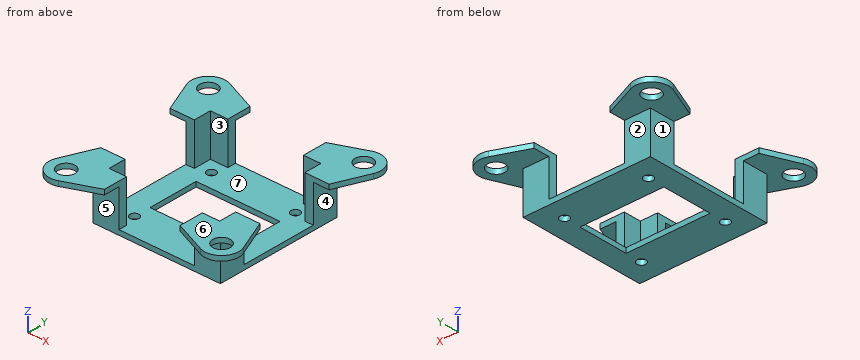
```python
from build123d import *

# Parameters (mm, degrees)
F0_W      = 39.5
F0_H      = 39.5
F0_R      = 1.625
F0_W_2    = 30
F0_H_2    = 18
F1_DEPTH  = 1.75
F2_W      = 45.5
F2_H      = 45.5
F2_W_2    = 39.5
F2_H_2    = 39.5
F3_DEPTH  = 15
F4_R      = 3.125
F4_W      = 39.5
F4_H      = 39.5
F5_DEPTH  = 1.75
F6_W      = 27.05052
F6_H      = 15
F7_DEPTH  = 25
F8_DEPTH  = 56.626
F9_W      = 27
F9_H      = 15
F10_DEPTH = 11.126
F11_DEPTH = 56.626


with BuildPart() as f1:
    # F0 (on Top) → F1 (new body)
    with BuildSketch(Plane.XY):
        Rectangle(F0_W, F0_H)
        with Locations((-15, -15)):
            Circle(F0_R, mode=Mode.SUBTRACT)
        with Locations((15, -15)):
            Circle(F0_R, mode=Mode.SUBTRACT)
        with Locations((-15, 15)):
            Circle(F0_R, mode=Mode.SUBTRACT)
        Rectangle(F0_W_2, F0_H_2, mode=Mode.SUBTRACT)
        with Locations((15, 15)):
            Circle(F0_R, mode=Mode.SUBTRACT)
    extrude(amount=F1_DEPTH)

    # F2 (on Top) → F3 (join)
    with BuildSketch(Plane.XY):
        Rectangle(F2_W, F2_H)
        Rectangle(F2_W_2, F2_H_2, mode=Mode.SUBTRACT)
    extrude(amount=F3_DEPTH)

    # F4 (on face) → F5 (join)
    with BuildSketch(Plane.XY.offset(15)):
        with BuildLine():
            Line((0, 22.75), (-25.380415, 33.39807))
            ThreePointArc((-25.380415, 33.39807), (-32.081029, 32.081029), (-33.39807, 25.380415))
            Line((-33.39807, 25.380415), (-22.75, 0))
            Line((-22.75, 0), (-33.39807, -25.380415))
            ThreePointArc((-33.39807, -25.380415), (-32.081029, -32.081029), (-25.380415, -33.39807))
            Line((-25.380415, -33.39807), (0, -22.75))
            Line((0, -22.75), (25.380415, -33.39807))
            ThreePointArc((25.380415, -33.39807), (32.081029, -32.081029), (33.39807, -25.380415))
            Line((33.39807, -25.380415), (22.75, 0))
            Line((22.75, 0), (33.39807, 25.380415))
            ThreePointArc((33.39807, 25.380415), (32.081029, 32.081029), (25.380415, 33.39807))
            Line((25.380415, 33.39807), (0, 22.75))
        make_face()
        with Locations((-27.75, -27.75)):
            Circle(F4_R, mode=Mode.SUBTRACT)
        with Locations((27.75, -27.75)):
            Circle(F4_R, mode=Mode.SUBTRACT)
        Rectangle(F4_W, F4_H, mode=Mode.SUBTRACT)
        with Locations((-27.75, 27.75)):
            Circle(F4_R, mode=Mode.SUBTRACT)
        with Locations((27.75, 27.75)):
            Circle(F4_R, mode=Mode.SUBTRACT)
    extrude(amount=F5_DEPTH)

    # F6 (on face) → F7 (cut)
    with BuildSketch(Plane.XZ.offset(22.75)):
        with Locations((0.02526, 9.25)):
            Rectangle(F6_W, F6_H)
    extrude(amount=F7_DEPTH, mode=Mode.SUBTRACT)

    # F6 (on face) → F8 (cut, through all)
    with BuildSketch(Plane.XZ.offset(22.75)):
        with Locations((0.02526, 9.25)):
            Rectangle(F6_W, F6_H)
    extrude(amount=-F8_DEPTH, mode=Mode.SUBTRACT)

    # F9 (on face) → F10 (cut, through all)
    with BuildSketch(Plane.YZ.offset(22.75)):
        with Locations((0, 9.25)):
            Rectangle(F9_W, F9_H)
    extrude(amount=F10_DEPTH, mode=Mode.SUBTRACT)

    # F9 (on face) → F11 (cut, through all)
    with BuildSketch(Plane.YZ.offset(22.75)):
        with Locations((0, 9.25)):
            Rectangle(F9_W, F9_H)
    extrude(amount=-F11_DEPTH, mode=Mode.SUBTRACT)


solid = f1.part
```
Geometry check sheet. Reference: the model listing, model coordinates, mm. Face numbers are marked on the shaded views. A direction names the side the tool comes from. Coordinates: 2 decimals unless noted, no trailing zeros. Order: outer loops, then holes, each group sorted by start corner. A loop starts at its lowest first (then second) coordinate and runs counter-clockwise, first axis right, second up.
Item 1: Depth check by flat-ended pin: pin 1 (5 mm diameter, centred on x = -17.5, z = 12, fed in from +Y); pin 2 (5 mm diameter, centred on x = 27.75, y = -27.75, fed in from +Z); pin 3 (2 mm diameter, centred on y = 14, z = 6, fed in from +X); pin 4 (4 mm diameter, centred on y = -15.5, z = 7, fed in from -X). Enter the tip coordinate at first touch or a pass-through.
Item 2: Tool access check on the marked faces 1, 2, 3 and 4. Record the directions out of +Z, -Z, +X, -X, +Y, -Y that give a thin tool (end or side, any length) a straight path to the whole face; none if there is none.
Item 3: Mould release check, pull along Y, two halves, no side actions. Record for the marked faces 5, 6 and 7: released by +Y, released by -Y, zero draft, split by the parting line, or undercut.
Item 4: Section check C-C (z = 10.25). Enter the section's corners in (x, y), plus the area to 3 significant figures.
Item 5: Section check D-D (y = 15). Enter the section's corners in (x, z) (3 decimals).
Item 6: Section check B-B (y = 5). Enter the section's corners in (x, z).
Item 7: Scan lines: line 1 along Y through (x, z) = (27.75, 16.2) (3 decimals); line 2 along X through (y, z) = (20.5, 14); line 3 along X through (y, z) = (-17, 14.75). Record each from-to range of solid material in increasing order.
Item 8: Section check A-A (x = 9). Enter the section's corners in (y, z), plus the area to 3 significant figures.
Check sheet entries:
1. pin 1: stops at y = 22.75
1. pin 2: passes through
1. pin 3: stops at x = 22.75
1. pin 4: stops at x = -22.75
2. face 1: -Z, -X, +Y, -Y
2. face 2: -Z, +X, -X, +Y
2. face 3: +Z
2. face 4: -Z, +X, +Y, -Y
3. face 5: released by -Y
3. face 6: zero draft
3. face 7: undercut
4. outline: (-22.75, -22.75) - (-13.5, -22.75) - (-13.5, -19.75) - (-19.75, -19.75) - (-19.75, -13.5) - (-22.75, -13.5) - close; (-22.75, 13.5) - (-19.75, 13.5) - (-19.75, 19.75) - (-13.5, 19.75) - (-13.5, 22.75) - (-22.75, 22.75) - close; (13.55, -22.75) - (22.75, -22.75) - (22.75, -13.5) - (19.75, -13.5) - (19.75, -19.75) - (13.55, -19.75) - close; (13.55, 19.75) - (19.75, 19.75) - (19.75, 13.5) - (22.75, 13.5) - (22.75, 22.75) - (13.55, 22.75) - close
4. area: 186 mm2
5. outline: (-29.043, 15) - (-22.75, 15) - (-22.75, 0) - (-16.625, 0) - (-16.625, 1.75) - (-19.75, 1.75) - (-19.75, 16.75) - (-29.043, 16.75) - close; (-13.375, 0) - (13.375, 0) - (13.375, 1.75) - (-13.375, 1.75) - close; (16.625, 0) - (22.75, 0) - (22.75, 15) - (29.043, 15) - (29.043, 16.75) - (19.75, 16.75) - (19.75, 1.75) - (16.625, 1.75) - close
6. outline: (-22.75, 0) - (-15, 0) - (-15, 1.75) - (-22.75, 1.75) - close; (15, 0) - (22.75, 0) - (22.75, 1.75) - (15, 1.75) - close
7. line 1: y = -33.875 to -30.875, -24.625 to -13.5, 13.5 to 24.625, 30.875 to 33.875
7. line 2: x = -22.75 to -13.5, 13.55 to 22.75
7. line 3: x = -22.75 to -19.75, 19.75 to 22.75
8. outline: (-22.75, 0) - (-9, 0) - (-9, 1.75) - (-22.75, 1.75) - close; (9, 0) - (22.75, 0) - (22.75, 1.75) - (9, 1.75) - close
8. area: 48.1 mm2
